```python
from build123d import *

# Parameters (mm, degrees)
SKETCH_1_W          = 60
SKETCH_1_H          = 40
EXTRUDE_1_DEPTH     = 1.5
SKETCH_3_R          = 2
CUT_EXTRUDE_1_DEPTH = 10
SKETCH_4_W          = 1
SKETCH_4_H          = 3
CUT_EXTRUDE_2_DEPTH = 10
FILLET_1_R          = 1


with BuildPart() as part:
    # 草图1 → 凸台-拉伸1 (new body)
    with BuildSketch(Plane.XY):
        Rectangle(SKETCH_1_W, SKETCH_1_H)
    extrude(amount=EXTRUDE_1_DEPTH)

    # 草图3 → 切除-拉伸1 (cut)
    with BuildSketch(Plane.XY.offset(1.5)):
        with Locations((-16, 0)):
            Circle(SKETCH_3_R)
        with Locations((16, 0)):
            Circle(SKETCH_3_R)
    extrude(amount=-CUT_EXTRUDE_1_DEPTH, mode=Mode.SUBTRACT)

    # 草图4 → 切除-拉伸2 (cut)
    with BuildSketch(Plane.XY.offset(1.5)):
        with Locations((-29.5, -10)):
            Rectangle(SKETCH_4_W, SKETCH_4_H)
        with Locations((29.5, -10)):
            Rectangle(SKETCH_4_W, SKETCH_4_H)
    extrude(amount=-CUT_EXTRUDE_2_DEPTH, mode=Mode.SUBTRACT)

    # 圆角1
    fillet_1_edges = [part.edges().sort_by_distance(p)[0] for p in [
        (-30, 20, 0.75),
        (30, 20, 0.75),
        (30, -20, 0.75),
        (-30, -20, 0.75),
    ]]
    fillet(fillet_1_edges, radius=FILLET_1_R)


solid = part.part
```
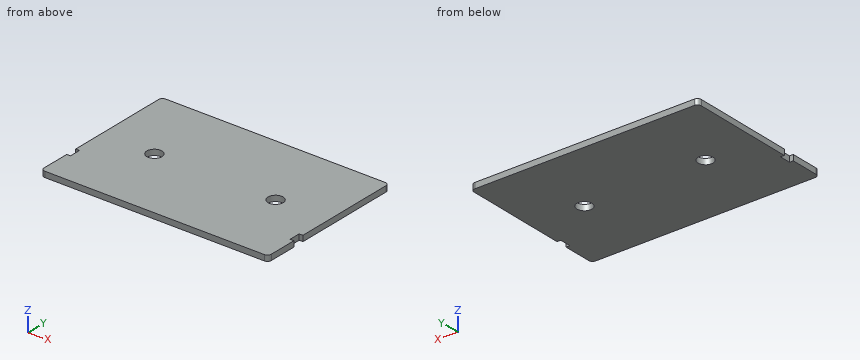
For this review, take the finished solid that the model builds, in its own axes (mm). Round coordinates to 2 decimals unless told otherwise and drop trailing zeros. Write each loop counter-clockwise with the first axis right and the second up, starting at its lowest first coordinate (ties: lowest second). Pieces come first, ordered by that corner, then holes. Notation, with made-up numbers: (12.5, -14.5) - (68.5, -14.5) arc R18 ccw to (68.5, 3.5) - close; hole circle Ø5 at (12, -2). An arc over 180 degrees is marked (long way). Answer as CSV lines item,"result". Start each with the question number.
(1) For pin 1 (0.8 mm diameter, centred on x = -29.5, z = 1, fed in from +Y) (3 decimals); pin 2 (0.8 mm diameter, centred on y = -10, z = 0.5, fed in from +X), all flat-tipped, find the tip position at first contact; note any pin that passes through.
(2) Add section B-B, the plane x = -16. State the section outline as (y, z) points, plus the area to 3 significant figures.
(3) Add section A-A, the plane y = 0. State the section outline as (x, z) points, plus the area to 3 significant figures.
(4) For line 1 (Y direction, x = -16, z = 1.25), list the stretches that pass through material, from the lowest coordinate up.
From the geometry:
1,pin 1,"stops at y = 19.995"
1,pin 2,"stops at x = 29"
2,outline,"(-20, 0) - (-2, 0) - (-2, 1.5) - (-20, 1.5) - close; (2, 0) - (20, 0) - (20, 1.5) - (2, 1.5) - close"
2,area,"54.0 mm²"
3,outline,"(-30, 0) - (-18, 0) - (-18, 1.5) - (-30, 1.5) - close; (-14, 0) - (14, 0) - (14, 1.5) - (-14, 1.5) - close; (18, 0) - (30, 0) - (30, 1.5) - (18, 1.5) - close"
3,area,"78.0 mm²"
4,line 1,"y = -20 to -2, 2 to 20"
